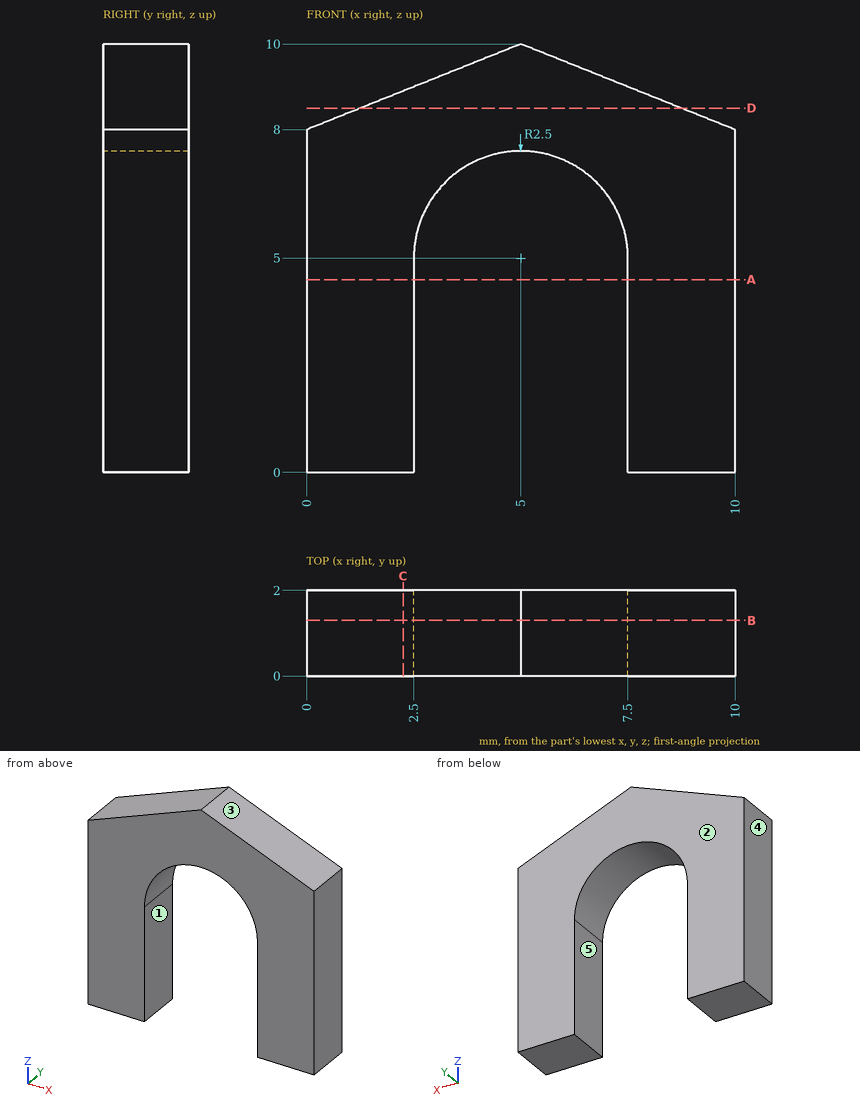
Can you work these out from the drawing? Everything is in mm from the part's minimum corner. A direction names the side the tool comes from. Round coordinates to 2 decimals unless told otherwise and drop trailing zeros. Loops run counter-clockwise (first coordinate to the right, second up) from the corner with the lowest first, then second, coordinate; pieces in that order, holes last. Notation, with made-up numbers: (18, 85) -> (76, 85) arc R19 ccw to (76, 100) -> close; hole circle Ø6 at (17.5, 19). An arc over 180 degrees is marked (long way). Answer in a Markdown table with one row per item.
Item 1: Suppose I cut it at D-D, the plane z = 8.5. List the corners of the cut face in (x, y) for me, plus the area to 3 significant figures.
Answer block:
| item | result |
|---|---|
| outline | (1.25, 0) -> (8.75, 0) -> (8.75, 2) -> (1.25, 2) -> close |
| area | 15.0 mm² |
Item 2: Suppose I cut it at A-A, the plane z = 4.5. List the corners of the cut face in (x, y) for me, plus the area to 3 significant figures.
Answer block:
| item | result |
|---|---|
| outline | (0, 0) -> (2.5, 0) -> (2.5, 2) -> (0, 2) -> close; (7.5, 0) -> (10, 0) -> (10, 2) -> (7.5, 2) -> close |
| area | 10.0 mm² |
Item 3: If I drill on probe 1 along X at (y, z) = (1.05, 4.75); probe 2 along X at (y, z) = (1.85, 6.5); probe 3 along Z at (x, y) = (8.5, 0.65), over which ranges is the centre line in solid material (lowest first)?
Answer block:
| item | result |
|---|---|
| probe 1 | 0 to 2.5, 7.5 to 10 |
| probe 2 | 0 to 3, 7 to 10 |
| probe 3 | 0 to 8.6 |
Item 4: Suppose I cut it at C-C, the plane x = 2.25. List the corners of the cut face in (y, z) for me, plus the area to 3 significant figures.
Answer block:
| item | result |
|---|---|
| outline | (0, 0) -> (2, 0) -> (2, 8.9) -> (0, 8.9) -> close |
| area | 17.8 mm² |
Item 5: Suppose I cut it at B-B, the plane y = 1.3. List the corners of the cut face in (x, z) for me, plus the area to 3 significant figures.
Answer block:
| item | result |
|---|---|
| outline | (0, 0) -> (2.5, 0) -> (2.5, 5) arc R2.5 cw to (7.5, 5) -> (7.5, 0) -> (10, 0) -> (10, 8) -> (5, 10) -> (0, 8) -> close |
| area | 55.2 mm² |
Item 6: On a 3-axis mill with a long thin cutter (end or side, diameter ignored), from which of +Z, -Z, +X, -X, +Y, -Y can I reach the whole of each face in a straight line? I mean the marked faces 4 and 5. Say none if no direction works.
Answer block:
| item | result |
|---|---|
| face 4 | +Z, -Z, -X, +Y, -Y |
| face 5 | -Z, +Y, -Y |
Item 7: We'd pull the mould along X, two halves only. Please class the marked faces 1, 2 and 3: released by +X, released by -X, zero draft, split by the parting line, or undercut.
Answer block:
| item | result |
|---|---|
| face 1 | undercut |
| face 2 | zero draft |
| face 3 | released by +X |
